CAD build for the part. Positions are in the model's coordinates, mm. Round coordinates to 2 decimals unless told otherwise and drop trailing zeros. Loops run counter-clockwise (first coordinate to the right, second up) from the corner with the lowest first, then second, coordinate; pieces in that order, holes last. Notation, with made-up numbers: (83.25, -31) - (140.25, -31) arc R23 cw to (140.25, -13) - close; hole circle Ø6 at (64.25, 48.5). An arc over 180 degrees is marked (long way). One line per question, with ' | ' between items.
```python
from build123d import *

# Parameters (mm, degrees)
F0_W     = 762
F0_H     = 203.2
F1_DEPTH = 25.4
F2_W     = 139.7
F2_H     = 88.9
F3_DEPTH = 50.8
F2_W_2   = 76.2
F2_H_2   = 152.4
F4_DEPTH = 50.8
F5_DEPTH = 50.8


with BuildPart() as f1:
    # F0 (on Front) → F1 (new body)
    with BuildSketch(Plane.XZ):
        with Locations((-1.348659, -86.213874)):
            Rectangle(F0_W, F0_H)
    extrude(amount=F1_DEPTH)

    # F2 (on face) → F3 (cut)
    with BuildSketch(Plane.XZ.offset(25.4)):
        with Locations((-210.898659, -79.863874)):
            Rectangle(F2_W, F2_H)
    extrude(amount=-F3_DEPTH, mode=Mode.SUBTRACT)

    # F2 (on face) → F4 (cut)
    with BuildSketch(Plane.XZ.offset(25.4)):
        with Locations((-1.348659, -111.613874)):
            Rectangle(F2_W_2, F2_H_2)
    extrude(amount=-F4_DEPTH, mode=Mode.SUBTRACT)

    # F2 (on face) → F5 (cut)
    with BuildSketch(Plane.XZ.offset(25.4)):
        with Locations((208.201341, -95.893279)):
            Rectangle(F2_W, F2_H)
    extrude(amount=-F5_DEPTH, mode=Mode.SUBTRACT)


solid = f1.part
```
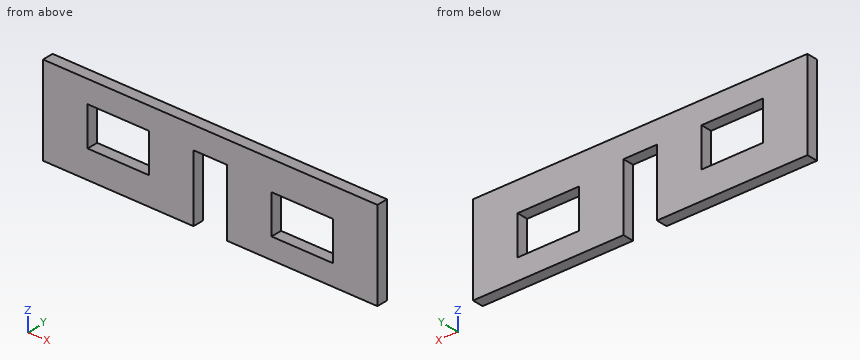
(1) Probe L1, parallel to X at y = -12, z = -46; L2, parallel to X at y = -9.75, z = -113; L3, parallel to Z at x = 164.5, y = -6. List the from-to ranges inside material, lowest first.
Results found:
L1: x = -382.35 to -280.75, -141.05 to -39.45, 36.75 to 379.65 | L2: x = -382.35 to -280.75, -141.05 to -39.45, 36.75 to 138.35, 278.05 to 379.65 | L3: z = -187.81 to -140.34, -51.44 to 15.39
(2) Cut at D-D, the plane z = -154. Write the cut outline in (x, y).
Results found:
outline: (-382.35, -25.4) - (-39.45, -25.4) - (-39.45, 0) - (-382.35, 0) - close; (36.75, -25.4) - (379.65, -25.4) - (379.65, 0) - (36.75, 0) - close
(3) Cut at C-C, the plane x = -272.5. Write the cut outline in (y, z).
Results found:
outline: (-25.4, -187.81) - (0, -187.81) - (0, -124.31) - (-25.4, -124.31) - close; (-25.4, -35.41) - (0, -35.41) - (0, 15.39) - (-25.4, 15.39) - close
(4) Cut at A-A, the plane z = -90. Write the cut outline in (x, y), then the cut area to 3 significant figures.
Results found:
outline: (-382.35, -25.4) - (-280.75, -25.4) - (-280.75, 0) - (-382.35, 0) - close; (-141.05, -25.4) - (-39.45, -25.4) - (-39.45, 0) - (-141.05, 0) - close; (36.75, -25.4) - (138.35, -25.4) - (138.35, 0) - (36.75, 0) - close; (278.05, -25.4) - (379.65, -25.4) - (379.65, 0) - (278.05, 0) - close | area: 10,300 mm²
(5) Drop a flat-ended pin along its axis: P1, Ø12.5, axis at x = -14, y = -14, coming from the -Z side. Give the stop position or say it passes through.
Results found:
P1: stops at z = -35.41
(6) Cut at B-B, the plane y = -14.5. Write the cut outline in (x, z), then the cut area to 3 significant figures.
Results found:
outline: (-382.35, -187.81) - (-39.45, -187.81) - (-39.45, -35.41) - (36.75, -35.41) - (36.75, -187.81) - (379.65, -187.81) - (379.65, 15.39) - (-382.35, 15.39) - close; hole (-280.75, -124.31) - (-141.05, -124.31) - (-141.05, -35.41) - (-280.75, -35.41) - close; hole (138.35, -140.34) - (278.05, -140.34) - (278.05, -51.44) - (138.35, -51.44) - close | area: 118,000 mm²
